```python
from build123d import *

# Parameters (mm, degrees)
F0_W     = 64
F0_H     = 17
F1_DEPTH = 2.5
F2_R     = 3
F3_DEPTH = 2.501


with BuildPart() as f1:
    # F0 (on Front) → F1 (new body)
    with BuildSketch(Plane.XZ):
        Rectangle(F0_W, F0_H)
    extrude(amount=F1_DEPTH)

    # F2 (on face) → F3 (cut, through all)
    with BuildSketch(Plane.XZ.offset(2.5)):
        with Locations((27, 0)):
            Circle(F2_R)
        with Locations((18, 0)):
            Circle(F2_R)
        with Locations((9, 0)):
            Circle(F2_R)
        Circle(F2_R)
        with Locations((-9, 0)):
            Circle(F2_R)
        with Locations((-18, 0)):
            Circle(F2_R)
        with Locations((-27, 0)):
            Circle(F2_R)
    extrude(amount=-F3_DEPTH, mode=Mode.SUBTRACT)


solid = f1.part
```
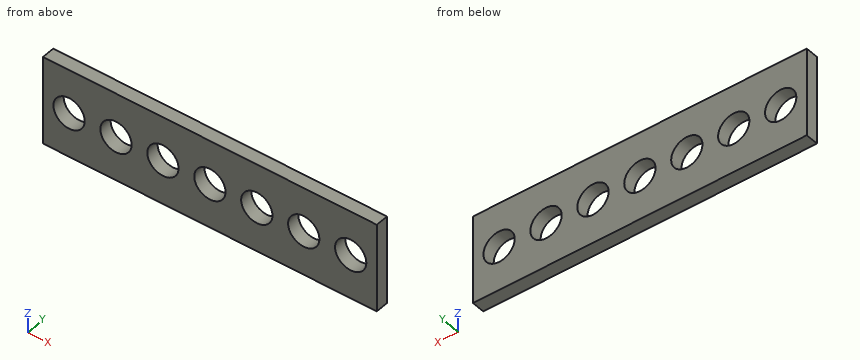
CAD build for the part. Positions are in the model's coordinates, mm. Coordinates: 2 decimals unless noted, no trailing zeros. Write each loop counter-clockwise with the first axis right and the second up, starting at its lowest first coordinate (ties: lowest second). Pieces come first, ordered by that corner, then holes. Notation, with made-up numbers: (-11, 7.25) -> (-4, 7.25) arc R17 cw to (-4, 28.25) -> close; hole circle Ø8 at (33.5, 80.5). An arc over 180 degrees is marked (long way). Return JSON: item names as keys, results as strings. Group by question number.
Q1. Flat gauge pin, fed straight in: pin 1 (5 mm diameter, centred on x = 0, z = 0, fed in from -Y). Where does the tip first touch, or does it go through?
Q2. Cut at C-C, the plane z = 1.25. State how many separate pieces and enclosed holes the cut face has, then the cut area to 3 significant figures.
Q3. Cut at B-B, the plane y = -0.5. Give the cut face in (x, z), then the cut area to 3 significant figures.
Q4. Cut at D-D, the plane x = -19. Give the cut face in (y, z).
Q5. Cut at A-A, the plane x = 0. Give the cut face in (y, z), then the cut area to 3 significant figures.
Q6. Drill centre lines: line 1 (Z direction, x = -18, y = -1.35); line 2 (Z direction, x = -29, y = -2.4). Where is each one in solid material? Low to high.
Returned:
{
 "1": {"pin 1": "passes through"},
 "2": {"separate pieces": "8", "enclosed holes": "0", "area": "64.5 mm2"},
 "3": {"outline": "(-32, -8.5) -> (32, -8.5) -> (32, 8.5) -> (-32, 8.5) -> close; hole circle Ø6 at (-27, 0); hole circle Ø6 at (-18, 0); hole circle Ø6 at (-9, 0); hole circle Ø6 at (0, 0); hole circle Ø6 at (9, 0); hole circle Ø6 at (18, 0); hole circle Ø6 at (27, 0)", "area": "890 mm2"},
 "4": {"outline": "(-2.5, -8.5) -> (0, -8.5) -> (0, -2.83) -> (-2.5, -2.83) -> close; (-2.5, 2.83) -> (0, 2.83) -> (0, 8.5) -> (-2.5, 8.5) -> close"},
 "5": {"outline": "(-2.5, -8.5) -> (0, -8.5) -> (0, -3) -> (-2.5, -3) -> close; (-2.5, 3) -> (0, 3) -> (0, 8.5) -> (-2.5, 8.5) -> close", "area": "27.5 mm2"},
 "6": {"line 1": "z = -8.5 to -3, 3 to 8.5", "line 2": "z = -8.5 to -2.24, 2.24 to 8.5"}
}
